Read the model definition and answer for the solid it produces. Units are mm, in the model's axes. Give positions to 0.01 mm unless a question says otherwise; leave off trailing zeros. Write each loop counter-clockwise with the first axis right and the second up, starting at its lowest first coordinate (ties: lowest second). Pieces come first, ordered by that corner, then holes. Notation, with made-up numbers: (-27, -37.75) -> (-23, -37.75) arc R14 cw to (-23, -21.75) -> close; hole circle Ø8 at (31, -19.5). An arc over 180 degrees is marked (long way). Write item = value, one per line.
from build123d import *

# Parameters (mm, degrees)
BOSS_EXTRUDE1_DEPTH = 5
SKETCH5_R           = 5
CUT_EXTRUDE4_DEPTH  = 5
SKETCH2_R           = 5
CUT_EXTRUDE5_DEPTH  = 5
BOSS_EXTRUDE2_DEPTH = 5


with BuildPart() as part:
    # Sketch1 → Boss-Extrude1 (new body)
    with BuildSketch(Plane(origin=(0, 0, 0), x_dir=(0, 0, -1), z_dir=(1, 0, 0))):
        Polygon((-95, 70), (-140, 70), (-140, 55), (-150, 55), (-150, 15), (-140, 15), (-140, 0), (-95, 0), (-95, 5), (-55, 5), (-55, 0), (-10, 0), (-10, 15), (0, 15), (0, 55), (-10, 55), (-10, 70), (-55, 70), (-55, 60), (-95, 60), align=None)
    extrude(amount=BOSS_EXTRUDE1_DEPTH)

    # Sketch5 → Cut-Extrude4 (cut)
    with BuildSketch(Plane.ZY):
        with Locations((37.111667647, 26.5)):
            Circle(SKETCH5_R)
        with Locations((72.52, 33)):
            Circle(SKETCH5_R)
    extrude(amount=-CUT_EXTRUDE4_DEPTH, mode=Mode.SUBTRACT)

    # Sketch2 → Cut-Extrude5 (cut)
    with BuildSketch(Plane(origin=(5, 0, 0), x_dir=(0, 0, -1), z_dir=(1, 0, 0))):
        with Locations((-108.52, 40)):
            Circle(SKETCH2_R)
    extrude(amount=-CUT_EXTRUDE5_DEPTH, mode=Mode.SUBTRACT)

    # Sketch6 → Boss-Extrude2 (add)
    with BuildSketch(Plane.ZY):
        Polygon((55, 0), (55, 5), (95, 5), (95, 0), (140, 0), (140, 15), (150, 15), (150, 55), (140, 55), (140, 70), (95, 70), (95, 60), (55, 60), (55, 70), (10, 70), (10, 55), (0, 55), (0, 15), (10, 15), (10, 0), align=None)
    extrude(amount=BOSS_EXTRUDE2_DEPTH)


solid = part.part
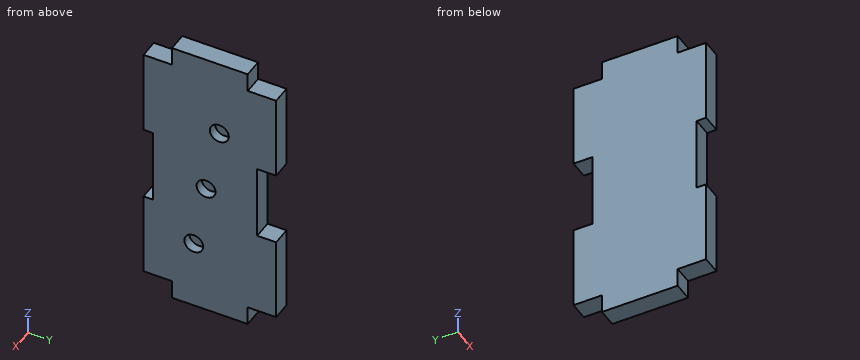
(1) The part is cut by section C-C on y = 26.5. Determine the outline of the cut face in (x, z).
Checks:
outline = (-5, 0) -> (5, 0) -> (5, 32.11) -> (0, 32.11) -> (0, 42.11) -> (5, 42.11) -> (5, 150) -> (-5, 150) -> close
(2) The part is cut by section D-D on z = 90. Determine the outline of the cut face in (x, y), plus the area to 3 significant figures.
Checks:
outline = (-5, 5) -> (5, 5) -> (5, 60) -> (-5, 60) -> close
area = 550 mm²
(3) Given P1, Ø3, axis at x = -1, z = 72, coming from the +Y side; P2, Ø3, axis at x = -0.5, y = 63, coming from the +Z side; P3, Ø8, axis at y = 42.5, z = 110.5, coming from the +X side; P4, Ø5, axis at x = 0.5, z = 144.5, coming from the +Y side, each flat-ended and moving along its own axis, determine where each tip first touches the part or whether it passes through.
Checks:
P1 = 60
P2 = 140
P3 = 5
P4 = 55
(4) Consider L1, parallel to Y at x = 1.25, z = 108.52; L2, parallel to Z at x = 4.25, y = 59.5; L3, parallel to X at y = 37.5, z = 111. Determine where each line is inside the solid, lowest interval first.
Checks:
L1 = 0 to 35, 45 to 70
L2 = 10 to 140
L3 = -5 to 0
(5) The part is cut by section A-A on x = 2.75. Determine the outline of the cut face in (y, z), plus the area to 3 significant figures.
Checks:
outline = (0, 10) -> (15, 10) -> (15, 0) -> (55, 0) -> (55, 10) -> (70, 10) -> (70, 55) -> (60, 55) -> (60, 95) -> (70, 95) -> (70, 140) -> (55, 140) -> (55, 150) -> (15, 150) -> (15, 140) -> (0, 140) -> (0, 95) -> (5, 95) -> (5, 55) -> (0, 55) -> close; hole circle Ø10 at (26.5, 37.11); hole circle Ø10 at (33, 72.52); hole circle Ø10 at (40, 108.52)
area = 9,060 mm²
(6) The part is cut by section B-B on z = 72.52. Determine the outline of the cut face in (x, y), plus the area to 3 significant figures.
Checks:
outline = (-5, 5) -> (5, 5) -> (5, 28) -> (0, 28) -> (0, 38) -> (5, 38) -> (5, 60) -> (-5, 60) -> close
area = 500 mm²
